from build123d import *

# Parameters (mm, degrees)
SKETCH2_R           = 4.5
BOSS_EXTRUDE1_DEPTH = 3.5
SKETCH2_3_R         = 4.5
SKETCH2_3_R_2       = 3.25
BOSS_EXTRUDE2_DEPTH = 1.25


with BuildPart() as part:
    # Sketch2 → Boss-Extrude1 (new body, symmetric)
    with BuildSketch(Plane(origin=(0, 0, 0), x_dir=(1, 0, 0), z_dir=(0, 1, 0))):
        with BuildLine():
            Line((-1.292919007, 6.625017769), (-0.973020228, 6.679500852))
            ThreePointArc((-0.973020228, 6.679500852), (-0.889453328, 6.659731402), (-0.845560152, 6.585923223))
            ThreePointArc((-0.845560152, 6.585923223), (-0.154320179, 5.998015112), (0.505801585, 6.620661002))
            ThreePointArc((0.505801585, 6.620661002), (0.544807056, 6.695768995), (0.625607777, 6.720945983))
            Line((0.625607777, 6.720945983), (0.947898066, 6.683096218))
            ThreePointArc((0.947898066, 6.683096218), (1.022510223, 6.640584052), (1.043831249, 6.557399487))
            ThreePointArc((1.043831249, 6.557399487), (1.541438291, 5.79856098), (2.350240104, 6.210007544))
            ThreePointArc((2.350240104, 6.210007544), (2.408825946, 6.271084025), (2.493446848, 6.272476974))
            Line((2.493446848, 6.272476974), (2.792018605, 6.145360723))
            ThreePointArc((2.792018605, 6.145360723), (2.851631383, 6.083549925), (2.848652958, 5.997728092))
            ThreePointArc((2.848652958, 5.997728092), (3.112313906, 5.129435773), (4.004271455, 5.296350057))
            ThreePointArc((4.004271455, 5.296350057), (4.077691391, 5.338446972), (4.159276992, 5.315943034))
            Line((4.159276992, 5.315943034), (4.409941708, 5.1098585))
            ThreePointArc((4.409941708, 5.1098585), (4.449725636, 5.033756613), (4.422689053, 4.952250287))
            ThreePointArc((4.422689053, 4.952250287), (4.431043665, 4.044848034), (5.333895854, 3.953707636))
            ThreePointArc((5.333895854, 3.953707636), (5.416201839, 3.973414544), (5.488142557, 3.928836854))
            Line((5.488142557, 3.928836854), (5.670592868, 3.66047978))
            ThreePointArc((5.670592868, 3.66047978), (5.687324888, 3.576252127), (5.638420492, 3.505664465))
            ThreePointArc((5.638420492, 3.505664465), (5.390791926, 2.632664613), (6.23139504, 2.290853186))
            ThreePointArc((6.23139504, 2.290853186), (6.315919132, 2.28657355), (6.372386759, 2.223533527))
            Line((6.372386759, 2.223533527), (6.471841626, 1.914644607))
            ThreePointArc((6.471841626, 1.914644607), (6.46416621, 1.829114811), (6.397355942, 1.775164406))
            ThreePointArc((6.397355942, 1.775164406), (5.913805593, 1.007292211), (6.624058967, 0.442501284))
            ThreePointArc((6.624058967, 0.442501284), (6.703953527, 0.414581815), (6.740373391, 0.338186587))
            Line((6.740373391, 0.338186587), (6.748775572, 0.013790165))
            ThreePointArc((6.748775572, 0.013790165), (6.717314536, -0.066112659), (6.638010968, -0.099055066))
            ThreePointArc((6.638010968, -0.099055066), (5.957713209, -0.699591165), (6.480076339, -1.441605591))
            ThreePointArc((6.480076339, -1.441605591), (6.548868784, -1.490903024), (6.562290365, -1.57446437))
            Line((6.562290365, -1.57446437), (6.478959166, -1.888087625))
            ThreePointArc((6.478959166, -1.888087625), (6.426261296, -1.955890225), (6.340889131, -1.965155837))
            ThreePointArc((6.340889131, -1.965155837), (5.51895764, -2.349703977), (5.811111772, -3.208828305))
            ThreePointArc((5.811111772, -3.208828305), (5.863228948, -3.275509917), (5.852564909, -3.359467737))
            Line((5.852564909, -3.359467737), (5.684251327, -3.636909935))
            ThreePointArc((5.684251327, -3.636909935), (5.614585891, -3.687119348), (5.530061474, -3.671957519))
            ThreePointArc((5.530061474, -3.671957519), (4.633084254, -3.809363897), (4.671360797, -4.715996984))
            ThreePointArc((4.671360797, -4.715996984), (4.702580479, -4.794660627), (4.668694758, -4.872213159))
            Line((4.668694758, -4.872213159), (4.429034558, -5.090997583))
            ThreePointArc((4.429034558, -5.090997583), (4.348045436, -5.11954614), (4.271216433, -5.081185191))
            ThreePointArc((4.271216433, -5.081185191), (3.371861242, -4.96031796), (3.153159258, -5.841009785))
            ThreePointArc((3.153159258, -5.841009785), (3.160952215, -5.925282599), (3.10659003, -5.990146997))
            Line((3.10659003, -5.990146997), (2.814999058, -6.132549034))
            ThreePointArc((2.814999058, -6.132549034), (2.729247506, -6.137123901), (2.666338146, -6.078671609))
            ThreePointArc((2.666338146, -6.078671609), (1.837465393, -5.709322713), (1.379502817, -6.492724861))
            ThreePointArc((1.379502817, -6.492724861), (1.363237709, -6.575779564), (1.292803162, -6.622700901))
            Line((1.292803162, -6.622700901), (0.972904383, -6.677183984))
            ThreePointArc((0.972904383, -6.677183984), (0.889337482, -6.657414534), (0.845444307, -6.583606355))
            ThreePointArc((0.845444307, -6.583606355), (0.154204334, -5.995698244), (-0.505917431, -6.618344134))
            ThreePointArc((-0.505917431, -6.618344134), (-0.544922901, -6.693452127), (-0.625723623, -6.718629115))
            Line((-0.625723623, -6.718629115), (-0.948013912, -6.68077935))
            ThreePointArc((-0.948013912, -6.68077935), (-1.022626068, -6.638267184), (-1.043947095, -6.555082619))
            ThreePointArc((-1.043947095, -6.555082619), (-1.541554137, -5.796244112), (-2.35035595, -6.207690676))
            ThreePointArc((-2.35035595, -6.207690676), (-2.408941792, -6.268767157), (-2.493562694, -6.270160106))
            Line((-2.493562694, -6.270160106), (-2.79213445, -6.143043855))
            ThreePointArc((-2.79213445, -6.143043855), (-2.851747229, -6.081233058), (-2.848768804, -5.995411224))
            ThreePointArc((-2.848768804, -5.995411224), (-3.112429751, -5.127118905), (-4.0043873, -5.294033189))
            ThreePointArc((-4.0043873, -5.294033189), (-4.077807237, -5.336130104), (-4.159392837, -5.313626166))
            Line((-4.159392837, -5.313626166), (-4.410057553, -5.107541632))
            ThreePointArc((-4.410057553, -5.107541632), (-4.449841481, -5.031439745), (-4.422804899, -4.949933419))
            ThreePointArc((-4.422804899, -4.949933419), (-4.43115951, -4.042531166), (-5.334011699, -3.951390768))
            ThreePointArc((-5.334011699, -3.951390768), (-5.416317684, -3.971097676), (-5.488258403, -3.926519986))
            Line((-5.488258403, -3.926519986), (-5.670708714, -3.658162912))
            ThreePointArc((-5.670708714, -3.658162912), (-5.687440734, -3.573935259), (-5.638536337, -3.503347597))
            ThreePointArc((-5.638536337, -3.503347597), (-5.390907771, -2.630347745), (-6.231510886, -2.288536318))
            ThreePointArc((-6.231510886, -2.288536318), (-6.316034978, -2.284256682), (-6.372502605, -2.221216659))
            Line((-6.372502605, -2.221216659), (-6.471957472, -1.912327739))
            ThreePointArc((-6.471957472, -1.912327739), (-6.464282055, -1.826797943), (-6.397471788, -1.772847538))
            ThreePointArc((-6.397471788, -1.772847538), (-5.913921439, -1.004975343), (-6.624174813, -0.440184416))
            ThreePointArc((-6.624174813, -0.440184416), (-6.704069372, -0.412264947), (-6.740489237, -0.335869719))
            Line((-6.740489237, -0.335869719), (-6.748891418, -0.011473297))
            ThreePointArc((-6.748891418, -0.011473297), (-6.717430382, 0.068429527), (-6.638126814, 0.101371934))
            ThreePointArc((-6.638126814, 0.101371934), (-5.957829055, 0.701908033), (-6.480192185, 1.443922459))
            ThreePointArc((-6.480192185, 1.443922459), (-6.54898463, 1.493219892), (-6.562406211, 1.576781238))
            Line((-6.562406211, 1.576781238), (-6.479075011, 1.890404493))
            ThreePointArc((-6.479075011, 1.890404493), (-6.426377141, 1.958207093), (-6.341004977, 1.967472704))
            ThreePointArc((-6.341004977, 1.967472704), (-5.519073486, 2.352020845), (-5.811227618, 3.211145173))
            ThreePointArc((-5.811227618, 3.211145173), (-5.863344793, 3.277826785), (-5.852680755, 3.361784605))
            Line((-5.852680755, 3.361784605), (-5.684367172, 3.639226803))
            ThreePointArc((-5.684367172, 3.639226803), (-5.614701737, 3.689436216), (-5.53017732, 3.674274387))
            ThreePointArc((-5.53017732, 3.674274387), (-4.633200099, 3.811680765), (-4.671476642, 4.718313851))
            ThreePointArc((-4.671476642, 4.718313851), (-4.702696325, 4.796977495), (-4.668810603, 4.874530027))
            Line((-4.668810603, 4.874530027), (-4.429150404, 5.093314451))
            ThreePointArc((-4.429150404, 5.093314451), (-4.348161282, 5.121863008), (-4.271332279, 5.083502059))
            ThreePointArc((-4.271332279, 5.083502059), (-3.371977088, 4.962634828), (-3.153275104, 5.843326652))
            ThreePointArc((-3.153275104, 5.843326652), (-3.161068061, 5.927599467), (-3.106705876, 5.992463865))
            Line((-3.106705876, 5.992463865), (-2.815114904, 6.134865902))
            ThreePointArc((-2.815114904, 6.134865902), (-2.729363352, 6.139440769), (-2.666453991, 6.080988477))
            ThreePointArc((-2.666453991, 6.080988477), (-1.837581239, 5.71163958), (-1.379618663, 6.495041729))
            ThreePointArc((-1.379618663, 6.495041729), (-1.363353555, 6.578096432), (-1.292919007, 6.625017769))
        make_face()
        Circle(SKETCH2_R, mode=Mode.SUBTRACT)
    extrude(amount=BOSS_EXTRUDE1_DEPTH, both=True)

    # Sketch2_3 → Boss-Extrude2 (add, symmetric)
    with BuildSketch(Plane(origin=(0, 0, 0), x_dir=(1, 0, 0), z_dir=(0, 1, 0))):
        Circle(SKETCH2_3_R)
        Circle(SKETCH2_3_R_2, mode=Mode.SUBTRACT)
    extrude(amount=BOSS_EXTRUDE2_DEPTH, both=True)


solid = part.part
Here's how the part is built. I have some questions about the finished solid (model axes, mm). A direction names the side the tool comes from. Coordinates: 2 decimals unless noted, no trailing zeros. Loops run counter-clockwise (first coordinate to the right, second up) from the corner with the lowest first, then second, coordinate; pieces in that order, holes last. Notation, with made-up numbers: (34.5, 25.5) -> (51.5, 25.5) arc R25 ccw to (51.5, 50.5) -> close; hole circle Ø10 at (30.5, 71). An arc over 180 degrees is marked (long way). Use one line per item in the form item = value. Start each with the question number.
(1) If we section it at B-B (z = -1): Please give me the cut outline in (x, y).
(2) Will these pins go through, and if not, where does the flat tip stop? pin 1 (1 mm diameter, centred on y = -2.5, z = 1.5, fed in from +X); pin 2 (3 mm diameter, centred on x = 5, y = -1.5, fed in from +Z).
(3) On a 3-axis mill with a long thin cutter (end or side, diameter ignored), from which of +Z, -Z, +X, -X, +Y, -Y can I reach the whole of each face in a straight line? I mean faces 1 (the face through (3, 1.25, 2)), 2 (the face through (3.383, 0.049, 4.953)), 3 (the face through (3, -1.25, 2)). Say none if no direction works.
(4) Please list where these lines run through material, in increasing order: line 1 along X through (y, z) = (-1.9, 0); line 2 along X through (y, z) = (0.7, 0); line 3 along Y through (x, z) = (2.5, -3).
(5) If we section it at A-A (x = 0): Please give me the cut outline in (y, z).
Verdict:
q1.outline = (-5.99, -3.5) -> (-4.39, -3.5) -> (-4.39, -1.25) -> (-3.09, -1.25) -> (-3.09, 1.25) -> (-4.39, 1.25) -> (-4.39, 3.5) -> (-5.99, 3.5) -> close; (3.09, -1.25) -> (4.39, -1.25) -> (4.39, -3.5) -> (5.92, -3.5) -> (5.92, 3.5) -> (4.39, 3.5) -> (4.39, 1.25) -> (3.09, 1.25) -> close
q2.pin_1 = 6.57
q2.pin_2 = 5.12
q3.face_1 = +Y
q3.face_2 = +Y, -Y
q3.face_3 = -Y
q4.line_1 = -6.75 to -4.5, 4.5 to 6.75
q4.line_2 = -6.75 to -3.25, 3.25 to 6.75
q4.line_3 = -1.25 to 1.25
q5.outline = (-3.5, -6.02) -> (3.5, -6.02) -> (3.5, -4.5) -> (1.25, -4.5) -> (1.25, -3.25) -> (-1.25, -3.25) -> (-1.25, -4.5) -> (-3.5, -4.5) -> close; (-3.5, 4.5) -> (-1.25, 4.5) -> (-1.25, 3.25) -> (1.25, 3.25) -> (1.25, 4.5) -> (3.5, 4.5) -> (3.5, 6.02) -> (-3.5, 6.02) -> close
